Verification items for the finished model (mm, model axes). Give positions to 0.01 mm unless a question says otherwise; leave off trailing zeros. Return JSON: item names as keys, results as strings. Group by question number.
(1) Cross-section at B-B on y = -72.5. State how many separate pieces and enclosed holes the cut face has, then the cut area to 3 significant figures.
(2) Depth check by flat-ended pin: pin 1 Ø0.9 at (y, z) = (-74, 1.5) entering from +X; pin 2 Ø0.9 at (x, z) = (107, 1.5) entering from -Y; pin 3 Ø1 at (y, z) = (-24.5, 1) entering from -X. Enter the tip coordinate at first touch or a pass-through.
(3) Thickness scan on line 1 along Y through (x, z) = (100.5, 1.55); line 2 along Y through (x, z) = (78, 1.75); line 3 along Y through (x, z) = (99, 0.35). Record the ranges inside material, lowest first.
from build123d import *

# Parameters (mm, degrees)
SKETCH_1_W      = 10
SKETCH_1_H      = 145
EXTRUDE_1_DEPTH = 3
FILLET_1_R      = 1.5


with BuildPart() as part:
    # 草图1 → 凸台-拉伸1 (new body)
    with BuildSketch(Plane.XY):
        Polygon((110.75, 71), (-110.75, 71), (-112.45, 71), (-112.45, 46), (-110.75, 46), (-110.75, 11), (-112.45, 11), (-112.45, -6), (-110.75, -6), (-110.75, -36), (-112.45, -36), (-112.45, -51), (-109, -51), (-109, -54), (-106, -54), (-106, -71), (-106, -86), (106, -86), (106, -71), (106, -54), (109, -54), (109, -51), (112.45, -51), (112.45, -36), (110.75, -36), (110.75, -6), (112.45, -6), (112.45, 11), (110.75, 11), (110.75, 46), (112.45, 46), (112.45, 71), align=None)
        with Locations((0, -8.5)):
            Rectangle(SKETCH_1_W, SKETCH_1_H, mode=Mode.SUBTRACT)
        with Locations((14, -8.5)):
            Rectangle(SKETCH_1_W, SKETCH_1_H, mode=Mode.SUBTRACT)
        with Locations((28, -8.5)):
            Rectangle(SKETCH_1_W, SKETCH_1_H, mode=Mode.SUBTRACT)
        with Locations((42, -8.5)):
            Rectangle(SKETCH_1_W, SKETCH_1_H, mode=Mode.SUBTRACT)
        with Locations((56, -8.5)):
            Rectangle(SKETCH_1_W, SKETCH_1_H, mode=Mode.SUBTRACT)
        with Locations((70, -8.5)):
            Rectangle(SKETCH_1_W, SKETCH_1_H, mode=Mode.SUBTRACT)
        with Locations((84, -8.5)):
            Rectangle(SKETCH_1_W, SKETCH_1_H, mode=Mode.SUBTRACT)
        with Locations((98, -8.5)):
            Rectangle(SKETCH_1_W, SKETCH_1_H, mode=Mode.SUBTRACT)
        with Locations((-14, -8.5)):
            Rectangle(SKETCH_1_W, SKETCH_1_H, mode=Mode.SUBTRACT)
        with Locations((-28, -8.5)):
            Rectangle(SKETCH_1_W, SKETCH_1_H, mode=Mode.SUBTRACT)
        with Locations((-42, -8.5)):
            Rectangle(SKETCH_1_W, SKETCH_1_H, mode=Mode.SUBTRACT)
        with Locations((-56, -8.5)):
            Rectangle(SKETCH_1_W, SKETCH_1_H, mode=Mode.SUBTRACT)
        with Locations((-70, -8.5)):
            Rectangle(SKETCH_1_W, SKETCH_1_H, mode=Mode.SUBTRACT)
        with Locations((-84, -8.5)):
            Rectangle(SKETCH_1_W, SKETCH_1_H, mode=Mode.SUBTRACT)
        with Locations((-98, -8.5)):
            Rectangle(SKETCH_1_W, SKETCH_1_H, mode=Mode.SUBTRACT)
    extrude(amount=EXTRUDE_1_DEPTH)

    # 圆角1
    fillet_1_edges = [part.edges().sort_by_distance(p)[0] for p in [
        (111.6, -6, 3),
        (111.6, -6, 0),
        (110.725, -51, 0),
        (110.725, -51, 3),
        (111.6, -36, 0),
        (111.6, -36, 3),
        (111.6, 11, 3),
        (111.6, 11, 0),
        (111.6, 46, 0),
        (111.6, 46, 3),
        (0, 71, 0),
        (0, 71, 3),
        (-111.6, 11, 0),
        (-111.6, 11, 3),
        (-111.6, -6, 0),
        (-111.6, -6, 3),
        (-111.6, 46, 0),
        (-111.6, 46, 3),
        (-111.6, -36, 0),
        (-111.6, -36, 3),
        (-110.725, -51, 0),
        (-110.725, -51, 3),
    ]]
    fillet(fillet_1_edges, radius=FILLET_1_R - 0.0001)  # a hair under: the kernel refuses the full size


solid = part.part
Verdict:
{
 "1": {"separate pieces": "16", "enclosed holes": "0", "area": "186 mm²"},
 "2": {"pin 1": "x = 106", "pin 2": "y = -54", "pin 3": "x = -110.75"},
 "3": {"line 1": "-86 to -81, 64 to 71", "line 2": "-86 to 70.98", "line 3": "-86 to -81, 64 to 70.46"}
}
